from build123d import *

# Parameters (mm, degrees)
SKETCH1_R                                           = 8
BOSS_EXTRUDE1_DEPTH                                 = 8
SKETCH3_W                                           = 44
SKETCH3_H                                           = 36
BOSS_EXTRUDE2_DEPTH                                 = 8
CSK_FOR_M6_COUNTERSUNK_FLAT_HEAD_SCREW1_D           = 6.6
CSK_FOR_M6_COUNTERSUNK_FLAT_HEAD_SCREW1_DEPTH       = 12
CSK_FOR_M6_COUNTERSUNK_FLAT_HEAD_SCREW1_CSINK_D     = 12.6
CSK_FOR_M6_COUNTERSUNK_FLAT_HEAD_SCREW1_CSINK_ANGLE = 90
CSK_FOR_M6_COUNTERSUNK_FLAT_HEAD_SCREW1_TIP         = 1.982840043
FILLET1_R                                           = 5
CHAMFER1_SIZE                                       = 0.5


with BuildPart() as part:
    # Sketch1 → Boss-Extrude1 (new body)
    with BuildSketch(Plane.XY):
        with BuildLine():
            Line((20, -18), (20, 18))
            Line((20, 18), (0, 18))
            ThreePointArc((0, 18), (-18, 0), (0, -18))
            Line((0, -18), (20, -18))
        make_face()
        Circle(SKETCH1_R, mode=Mode.SUBTRACT)
    extrude(amount=BOSS_EXTRUDE1_DEPTH)

    # Sketch3 → Boss-Extrude2 (add)
    with BuildSketch(Plane(origin=(20, 0, 0), x_dir=(0, 0, -1), z_dir=(1, 0, 0))):
        with Locations((-4, 0)):
            Rectangle(SKETCH3_W, SKETCH3_H)
    extrude(amount=BOSS_EXTRUDE2_DEPTH)

    # CSK for M6 Countersunk Flat Head Screw1
    with Locations(Plane.ZY.offset(-20)):
        with Locations((-9, 9), (-9, -9)):
            CounterSinkHole(CSK_FOR_M6_COUNTERSUNK_FLAT_HEAD_SCREW1_D / 2, CSK_FOR_M6_COUNTERSUNK_FLAT_HEAD_SCREW1_CSINK_D / 2, depth=CSK_FOR_M6_COUNTERSUNK_FLAT_HEAD_SCREW1_DEPTH, counter_sink_angle=CSK_FOR_M6_COUNTERSUNK_FLAT_HEAD_SCREW1_CSINK_ANGLE)
            with Locations((0, 0, -(CSK_FOR_M6_COUNTERSUNK_FLAT_HEAD_SCREW1_DEPTH + CSK_FOR_M6_COUNTERSUNK_FLAT_HEAD_SCREW1_TIP / 2))):  # 118° drill point
                Cone(0, CSK_FOR_M6_COUNTERSUNK_FLAT_HEAD_SCREW1_D / 2, CSK_FOR_M6_COUNTERSUNK_FLAT_HEAD_SCREW1_TIP, mode=Mode.SUBTRACT)

    # Fillet1
    fillet1_edges = [part.edges().sort_by_distance(p)[0] for p in [
        (24, -18, -18),
        (24, 18, -18),
    ]]
    fillet(fillet1_edges, radius=FILLET1_R)

    # Mirror1: part across plane


with BuildPart() as part_1:
    add(part.part)
    add(part.part.mirror(Plane(origin=(28, -18, 26), x_dir=(1, 0, 0), z_dir=(0, 0, -1))))

    # Chamfer1
    chamfer1_edges = [part_1.edges().sort_by_distance(p)[0] for p in [
        (-8, 0, 0),
        (-8, 0, 8),
        (20, 0, 8),
        (10, 18, 8),
        (20, 18, 26),
        (20, -18, 26),
        (20, -18, -6.5),
        (20, 0, -18),
        (20, 18, -6.5),
        (20, 16.535533906, -16.535533906),
        (-18, 0, 8),
        (10, 18, 0),
        (20, -16.535533906, -16.535533906),
        (20, 0, 0),
        (10, -18, 0),
        (-18, 0, 0),
        (-8, 0, 44),
        (-18, 0, 52),
        (10, -18, 52),
        (20, 0, 52),
        (10, 18, 52),
        (-18, 0, 44),
        (10, -18, 44),
        (10, 18, 44),
        (-8, 0, 52),
        (20, 0, 70),
        (20, 18, 58.5),
        (20, -18, 58.5),
        (20, 0, 44),
        (20, -16.535533906, 68.535533906),
        (20, 16.535533906, 68.535533906),
        (10, -18, 8),
    ]]
    chamfer(chamfer1_edges, length=CHAMFER1_SIZE)


solid = part_1.part
Geometry check sheet. Reference: the model listing, model coordinates, mm. A direction names the side the tool comes from. Coordinates: 2 decimals unless noted, no trailing zeros. Order: outer loops, then holes, each group sorted by start corner. A loop starts at its lowest first (then second) coordinate and runs counter-clockwise, first axis right, second up. Notation, with made-up numbers: M -27.5,68 L -9.5,68 A34 ccw -9.5,101 Z; hole C 59,26 d9. An arc over 180 degrees is marked long. Use CSV: the item, a comma, the result in double quotes.
Item 1: Thickness scan on line 1 along Y through (x, z) = (25, 61); line 2 along Z through (x, y) = (26.3, -9); line 3 along Z through (x, y) = (20.5, 11). Record the ranges inside material, lowest first.
Returned:
line 1,"y = -18 to -12.3, -5.7 to 5.7, 12.3 to 18"
line 2,"z = -18 to -12.3, -5.7 to 57.7, 64.3 to 70"
line 3,"z = -18 to -14.44, -3.56 to 55.56, 66.44 to 70"
Item 2: Mould release check, pull along Y, two halves, no side actions. Record for faces 6 (the conical face through (-17.638, 0.388, 44.142)), 7 (the conical face through (22.854, -8.849, -5.558)), 8 (the flat face through (9, 0, 0)): pulls with the +Y half, pulls with the -Y half, needs draft (parallel to the pull), parting line crosses it, or undercut.
Returned:
face 6,"parting line crosses it"
face 7,"undercut"
face 8,"needs draft"
Item 3: Tool access check on faces 1 (the conical face through (-17.638, 0.388, 7.858)), 2 (the flat face through (9, 0, 8)), 3 (the cylindrical face through (-1.73, -7.81, 48.05)), 4 (the flat face through (20, 0, 61)), 5 (the cylindrical face through (25.5, -8.9, 57.7)). Record the directions out of +Z, -Z, +X, -X, +Y, -Y that give a thin tool (end or side, any length) a straight path to the whole face; none if there is none.
Returned:
face 1,"-X"
face 2,"-X, +Y, -Y"
face 3,"+Z, -Z"
face 4,"+Z, -X, +Y, -Y"
face 5,"+X, -X"
Item 4: Cross-section at D-D on y = 0. Give the number of separate pieces and of enclosed holes in the cut face, then the cut area to 3 significant figures.
Returned:
separate pieces,"3"
enclosed holes,"0"
area,"1,050 mm2"
Item 5: Gauge pin test, flat ends, axial feed: pin 1 Ø6 at (y, z) = (-9, 61) entering from +X; pin 2 Ø7.5 at (y, z) = (9, 61) entering from -X; pin 3 Ø10.5 at (x, y) = (-5.5, 1.5) entering from +Z; pin 4 Ø5 at (y, z) = (-2.5, -3.5) entering from -X. Record the tip position at first contact, or that the pin passes through.
Returned:
pin 1,"passes through"
pin 2,"stops at x = 22.55"
pin 3,"stops at z = 52"
pin 4,"stops at x = 20"
Item 6: Cross-section at A-A on x = 12.5. Record the cut outline in (y, z).
Returned:
outline,"M -18,0.5 L -17.5,0 L 17.5,0 L 18,0.5 L 18,7.5 L 17.5,8 L -17.5,8 L -18,7.5 Z; M -18,44.5 L -17.5,44 L 17.5,44 L 18,44.5 L 18,51.5 L 17.5,52 L -17.5,52 L -18,51.5 Z"
Item 7: Cross-section at C-C on z = 49.5. Record the cut outline in (x, y).
Returned:
outline,"M 0,-18 L 28,-18 L 28,18 L 0,18 A18 ccw Z; hole C 0,0 d16"
Item 8: Cross-section at B-B on z = -9. Record the cut outline in (x, y), then the cut area to 3 significant figures.
Returned:
outline,"M 20,-17.5 L 20.5,-18 L 28,-18 L 28,-12.3 L 23,-12.3 L 20,-15.3 Z; M 20,-2.7 L 23,-5.7 L 28,-5.7 L 28,5.7 L 23,5.7 L 20,2.7 Z; M 20,15.3 L 23,12.3 L 28,12.3 L 28,18 L 20.5,18 L 20,17.5 Z"
area,"164 mm2"
